from build123d import *

# Parameters (mm, degrees)
SKETCH1_R               = 2.5
BOSS_EXTRUDE1_DEPTH     = 3
SKETCH1_3_R             = 2.5
BOSS_EXTRUDE2_DEPTH     = 42
SKETCH2_R               = 1.5
CUT_EXTRUDE1_DEPTH      = 147
BOSS_EXTRUDE3_START     = 23
SKETCH3_R               = 5
BOSS_EXTRUDE3_DEPTH     = 2
SKETCH4_R               = 4
BOSS_EXTRUDE4_DEPTH     = 17
SKETCH2_3_R             = 1.5
CUT_EXTRUDE2_DEPTH      = 101
CUT_EXTRUDE2_DEPTH_BACK = 130


with BuildPart() as part:
    # Sketch1 → Boss-Extrude1 (new body)
    with BuildSketch(Plane(origin=(0, 0, 0), x_dir=(1, 0, 0), z_dir=(0, 1, 0))):
        with BuildLine():
            ThreePointArc((-40, 36), (-38.828427125, 38.828427125), (-36, 40))
            Line((-36, 40), (36, 40))
            ThreePointArc((36, 40), (38.828427125, 38.828427125), (40, 36))
            Line((40, 36), (40, -36))
            ThreePointArc((40, -36), (38.828427125, -38.828427125), (36, -40))
            Line((36, -40), (-36, -40))
            ThreePointArc((-36, -40), (-38.828427125, -38.828427125), (-40, -36))
            Line((-40, -36), (-40, 36))
        make_face()
        with Locations((35, 34)):
            Circle(SKETCH1_R, mode=Mode.SUBTRACT)
        with Locations((35, -34)):
            Circle(SKETCH1_R, mode=Mode.SUBTRACT)
        with Locations((-35, -34)):
            Circle(SKETCH1_R, mode=Mode.SUBTRACT)
        with Locations((-35, 34)):
            Circle(SKETCH1_R, mode=Mode.SUBTRACT)
        with Locations((-35, 34)):
            Circle(SKETCH1_R)
        with Locations((35, 34)):
            Circle(SKETCH1_R)
        with Locations((-35, -34)):
            Circle(SKETCH1_R)
        with Locations((35, -34)):
            Circle(SKETCH1_R)
    extrude(amount=BOSS_EXTRUDE1_DEPTH)

    # Sketch1<3> → Boss-Extrude2 (add)
    with BuildSketch(Plane(origin=(0, 0, 0), x_dir=(1, 0, 0), z_dir=(0, 1, 0))):
        with Locations((-35, 34)):
            Circle(SKETCH1_3_R)
        with Locations((-35, -34)):
            Circle(SKETCH1_3_R)
        with Locations((35, -34)):
            Circle(SKETCH1_3_R)
        with Locations((35, 34)):
            Circle(SKETCH1_3_R)
    extrude(amount=-BOSS_EXTRUDE2_DEPTH)

    # Sketch2 → Cut-Extrude1 (cut)
    with BuildSketch(Plane.ZY.offset(37.5)):
        with Locations((-34, -38)):
            Circle(SKETCH2_R)
        with Locations((34, -38)):
            Circle(SKETCH2_R)
    extrude(amount=-CUT_EXTRUDE1_DEPTH, mode=Mode.SUBTRACT)

    # Sketch3 → Boss-Extrude3 (add)
    with BuildSketch(Plane.XZ.offset(BOSS_EXTRUDE3_START)):
        with Locations((35, 34)):
            Circle(SKETCH3_R)
        with Locations((-35, 34)):
            Circle(SKETCH3_R)
        with Locations((-35, -34)):
            Circle(SKETCH3_R)
        with Locations((35, -34)):
            Circle(SKETCH3_R)
    extrude(amount=BOSS_EXTRUDE3_DEPTH)

    # Sketch4 → Boss-Extrude4 (add)
    with BuildSketch(Plane.XZ.offset(25)):
        with Locations((-35, 34)):
            Circle(SKETCH4_R)
        with Locations((35, 34)):
            Circle(SKETCH4_R)
        with Locations((-35, -34)):
            Circle(SKETCH4_R)
        with Locations((35, -34)):
            Circle(SKETCH4_R)
    extrude(amount=BOSS_EXTRUDE4_DEPTH)

    # Sketch2<3> → Cut-Extrude2 (cut, two sides)
    with BuildSketch(Plane.ZY.offset(37.5)) as cut_extrude2_sk:
        with Locations((-34, -38)):
            Circle(SKETCH2_3_R)
        with Locations((34, -38)):
            Circle(SKETCH2_3_R)
    extrude(amount=CUT_EXTRUDE2_DEPTH, mode=Mode.SUBTRACT)
    extrude(cut_extrude2_sk.sketch, amount=-CUT_EXTRUDE2_DEPTH_BACK, mode=Mode.SUBTRACT)


solid = part.part
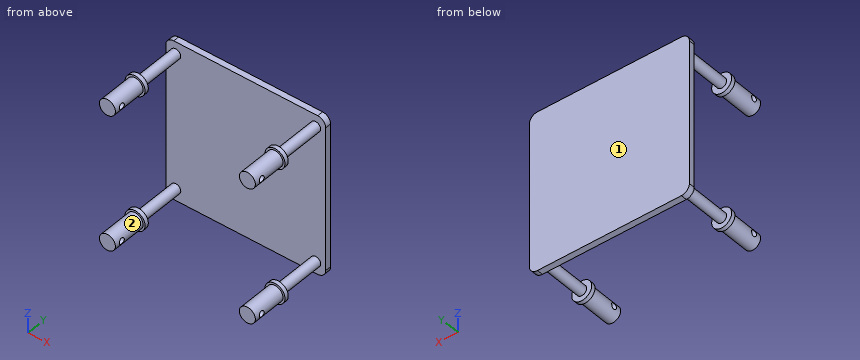
Geometry check sheet. Reference: the model listing, model coordinates, mm. Face numbers are marked on the shaded views. Round coordinates to 2 decimals unless told otherwise and drop trailing zeros. Write each loop counter-clockwise with the first axis right and the second up, starting at its lowest first coordinate (ties: lowest second). Pieces come first, ordered by that corner, then holes. Notation, with made-up numbers: (27, -30) -> (84, -30) arc R10 cw to (84, -21) -> close; hole circle Ø11 at (-36, -9). An arc over 180 degrees is marked (long way). One line per item, written item: value. Start each with the question number.
(1) Cross-section at D-D, the plane z = 4.5. Record the cut outline in (x, y), and give its area (3 significant figures).
(2) Go/stop test with flat-tipped pins: pin 1 Ø5 at (y, z) = (-38, -34) entering from +X; pin 2 Ø4 at (y, z) = (-38, 34) entering from -X; pin 3 Ø8 at (x, z) = (3.5, 5) entering from -Y; pin 4 Ø1.8 at (y, z) = (-38, -34) entering from -X (3 decimals). Record where each tip stops, or that it passes through.
(3) Scan lines: line 1 (Z direction, x = 35, y = -34); line 2 (X direction, y = -8.5, z = 34); line 3 (Z direction, x = -35, y = -38). Record each from-to range of solid material in increasing order. Write a range as [from, to].
(4) Cross-section at C-C, the plane y = -38. Record the cut outline in (x, z), and give its area (3 significant figures).
(5) Draft check along Z on the marked faces 1 and 2. Enter one of: +Z half, -Z half, draft (parallel to the pull), parting line (faces both ways), or undercut.
(6) Cross-section at B-B, the plane y = -4.5. Record the cut outline in (x, z).
(7) Cross-section at A-A, the plane x = -35. Give the number of separate pieces and of enclosed holes in the cut face, and give its area (3 significant figures).
Answer:
1. outline: (-40, 0) -> (40, 0) -> (40, 3) -> (-40, 3) -> close
1. area: 240 mm²
2. pin 1: x = 39
2. pin 2: x = -39
2. pin 3: y = 0
2. pin 4: through
3. line 1: [-38, -30], [30, 38]
3. line 2: [-37.5, -32.5], [32.5, 37.5]
3. line 3: [-38, -35.5], [-32.5, -30], [30, 32.5], [35.5, 38]
4. outline: (-38.71, -35.5) arc R4 ccw to (-31.29, -35.5) -> close; (-38.71, -32.5) -> (-31.29, -32.5) arc R4 ccw to start; (-38.71, 32.5) arc R4 ccw to (-31.29, 32.5) -> close; (-38.71, 35.5) -> (-31.29, 35.5) arc R4 ccw to start; (31.29, -35.5) arc R4 ccw to (38.71, -35.5) -> close; (31.29, -32.5) -> (38.71, -32.5) arc R4 ccw to start; (31.29, 32.5) arc R4 ccw to (38.71, 32.5) -> close; (31.29, 35.5) -> (38.71, 35.5) arc R4 ccw to start
4. area: 107 mm²
5. face 1: draft
5. face 2: undercut
6. outline: circle Ø5 at (-35, -34); circle Ø5 at (-35, 34); circle Ø5 at (35, -34); circle Ø5 at (35, 34)
7. separate pieces: 1
7. enclosed holes: 2
7. area: 768 mm²
